from build123d import *

# Parameters (mm, degrees)
IZIM1_R                     = 16
Y_KSEKLIK_EKSTR_ZYON1_DEPTH = 20
PAH2_SIZE                   = 3
PAH3_SIZE                   = 3
IZIM2_R                     = 9
Y_KSEKLIK_EKSTR_ZYON2_DEPTH = 135
IZIM3_R                     = 3
KES_EKSTR_ZYON1_DEPTH       = 149.967052528


with BuildPart() as part:
    # Çizim1 → Yükseklik-Ekstrüzyon1 (new body)
    with BuildSketch(Plane.XY):
        with Locations((-35.687497372, 19.980346779)):
            Circle(IZIM1_R)
    extrude(amount=Y_KSEKLIK_EKSTR_ZYON1_DEPTH)

    # Pah2
    pah2_edges = [part.edges().sort_by_distance(p)[0] for p in [
        (-51.687497372, 19.980346779, 20),
    ]]
    chamfer(pah2_edges, length=PAH2_SIZE)

    # Pah3
    pah3_edges = [part.edges().sort_by_distance(p)[0] for p in [
        (-51.687497372, 19.980346779, 0),
    ]]
    chamfer(pah3_edges, length=PAH3_SIZE)

    # Çizim2 → Yükseklik-Ekstrüzyon2 (add)
    with BuildSketch(Plane(origin=(0, 0, 0), x_dir=(-1, 0, 0), z_dir=(0, 0, -1))):
        with Locations((35.687497372, 19.980346779)):
            Circle(IZIM2_R)
    extrude(amount=Y_KSEKLIK_EKSTR_ZYON2_DEPTH)

    # Çizim3 → Kes-Ekstrüzyon1 (cut, through all)
    with BuildSketch(Plane(origin=(0, 0, 0), x_dir=(0, 0, -1), z_dir=(1, 0, 0))):
        with Locations((-10, 19.980346779)):
            Circle(IZIM3_R)
    extrude(amount=-KES_EKSTR_ZYON1_DEPTH, mode=Mode.SUBTRACT)


solid = part.part
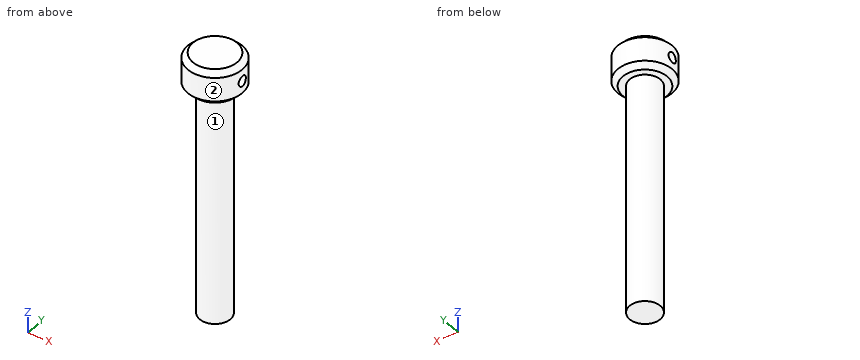
Input: part model. Units: mm. Frame: model coordinates. Face numbers are marked on the shaded views. A direction names the side the tool comes from. Coordinates: 2 decimals unless noted, no trailing zeros. Order: outer loops, then holes, each group sorted by start corner. A loop starts at its lowest first (then second) coordinate and runs counter-clockwise, first axis right, second up. Notation, with made-up numbers: M 65.5,82 L 92.5,82 A20 ccw 92.5,90 Z; hole C 4,-18.75 d11. An arc over 180 degrees is marked long. Answer in a Markdown table with one row per item.
(1) Section query A-A, the plane z = 10. Output: boundary loops of the cut face in (x, y).
Numbers:
| item | result |
|---|---|
| outline | M -51.4,16.98 A16 ccw -19.97,16.98 Z; M -51.4,22.98 L -19.97,22.98 A16 ccw Z |
(2) Access query for the marked faces 1 and 2. Directions: +Z, -Z, +X, -X, +Y, -Y. A direction counts if a zero-diameter tool reaches every point of the face in a straight line with its end or side. Return the directions, or none.
Numbers:
| item | result |
|---|---|
| face 1 | -Z |
| face 2 | +Z, -Z |
(3) Section query B-B, the plane z = -54. Output: boundary loops of the cut face in (x, y).
Numbers:
| item | result |
|---|---|
| outline | C -35.69,19.98 d18 |
(4) Contact query for flat-ended pins moving along their axis: pin 1 Ø10 at (x, z) = (-25, -80.5) entering from -Y; pin 2 Ø6 at (y, z) = (12, -10) entering from -X; pin 3 Ø5 at (x, y) = (-25, 13) entering from -Z. Output: stop coordinate, or through.
Numbers:
| item | result |
|---|---|
| pin 1 | stops at y = 13.01 |
| pin 2 | stops at x = -43.18 |
| pin 3 | stops at z = 0 |
(5) Material intervals for line 1 (Z direction, x = -42, y = 26.5); line 2 (Z direction, x = -29.5, y = 21); line 3 (Y direction, x = -42, z = 10), sorted ascending. Write a range as [from, to].
Numbers:
| item | result |
|---|---|
| line 1 | z = [0, 20] |
| line 2 | z = [-135, 7.18], [12.82, 20] |
| line 3 | y = [5.28, 16.98], [22.98, 34.68] |
